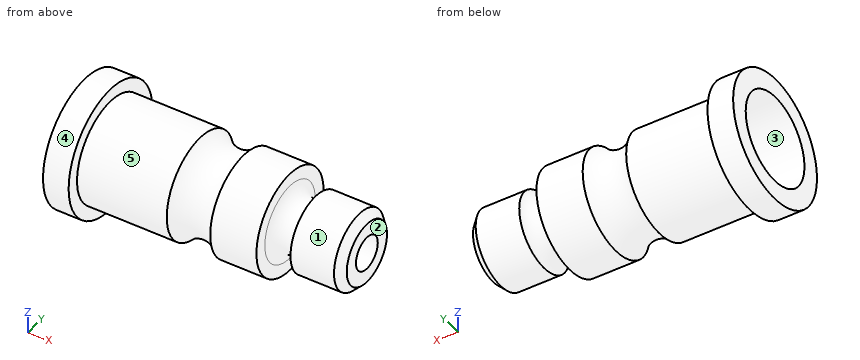
Autodesk Inventor part; units mm, degrees
ref_plane "YZ Plane" through (0, 0, 0) normal (1, 0, 0) x (0, 1, 0)
ref_plane "XZ Plane" through (0, 0, 0) normal (0, 1, 0) x (-1, 0, 0)
ref_plane "XY Plane" through (0, 0, 0) normal (0, 0, 1) x (1, 0, 0)
sketch "Skizze1" plane through (0, 0, 0) normal (0, 0, 1) x (1, 0, 0)
  line L0 (0, -1.0072) -> (0, 6.0435)
  line L1 (-2.2, 0) -> (13.2, 0)
  line L2 (0, 2.5) -> (0, 1.75)
  line L3 (0, 2.5) -> (1, 2.5)
  line L4 (1, 2.5) -> (1, 2)
  line L5 (1, 2) -> (4.5, 2)
  line L6 (0, 1.75) -> (4, 1.75)
  arc A0 (4.5, 2) -> (6.1971, 2) centre (5.3485, 2.7) ccw
  line L7 (6.1971, 2) -> (8, 2)
  line L8 (8, 2) -> (8, 1.5)
  arc A1 (8, 1.5) -> (9, 1.5) centre (8.5, 1.5) ccw
  line L9 (9, 1.5) -> (11, 1.5)
  line L10 (11, 1.5) -> (11, 0.65)
  line L11 (11, 0.65) -> (4.923, 0.65)
  line L12 (4.923, 0.65) -> (4, 1.75)
  line L13 (5.3485, 5.0362) -> (5.3485, 0.3638) construction
  point P0 (0, 0)
  dimension "d0" = 4
  dimension "d1" = 5
  dimension "d2" = 3.5
  dimension "d3" = 4
  dimension "d4" = 1.3
  dimension "d6" = 6.5
  dimension "d7" = 0.5
  dimension "d8" = 3
  dimension "d9" = 3
  dimension "d10" = 11
  dimension "d11" = 1
  dimension "d13" = 3.2
  dimension "d14" = 1.1
  dimension "d15" = 130
revolve "Umdrehung1" add sketch "Skizze1" angle 360 about axis through (-10, 0, 0) along (1, 0, 0)
thread "Gewinde1"
chamfer "Fase1" distance 0.3 angle 45 1 edges at (11, -1.5, 0)
properties part number "Öler"
Design review of the part built by this model. Coordinates are the model's own, in mm. Face numbers are marked on the shaded views. A direction names the side the tool comes from. Round coordinates to 2 decimals unless told otherwise and drop trailing zeros. Write each loop counter-clockwise with the first axis right and the second up, starting at its lowest first coordinate (ties: lowest second). Pieces come first, ordered by that corner, then holes.
Item 1: The part is to be moulded in two halves that separate along Z. For the marked faces 1, 2 and 3, say which applies: +Z half, -Z half, draft (parallel to the pull), parting line (faces both ways), or undercut.
Item 2: For the marked faces 4 and 5, list the 3-axis set-ups (+Z, -Z, +X, -X, +Y, -Y) from which the entire face can be reached by the end or side of a thin tool; tool diameter is ignored.
Item 3: We need section D-D on x = 9.5. Write out the cut boundary in (y, z), and give its area (3 significant figures).
Item 4: For probe 1 along Z at (x, y) = (1.4, 0); probe 2 along Z at (x, y) = (9.75, 0); probe 3 along X at (y, z) = (0.55, 2.15), list the stretches that pass through material, from the lowest coordinate up.
Item 5: Clearance check with flat-ended pins moving along their axes: pin 1 Ø2 at (x, z) = (3.5, 0.5) entering from -Y; pin 2 Ø1.5 at (x, y) = (3, 0) entering from -Z; pin 3 Ø2 at (y, z) = (0, 0) entering from -X. State where each tip first meets the part, or that it passes through.
Item 6: We need section A-A on y = 0. Write out the cut boundary in (x, z).
Item 7: We need section C-C on x = 7. Write out the cut boundary in (y, z), and give its area (3 significant figures).
Returned:
1. face 1: parting line
1. face 2: draft
1. face 3: undercut
2. face 4: +X, -X
2. face 5: +X
3. outline: circle Ø3 at (0, 0); hole circle Ø1.3 at (0, 0)
3. area: 5.74 mm2
4. probe 1: z = -2 to -1.75, 1.75 to 2
4. probe 2: z = -1.5 to -0.65, 0.65 to 1.5
4. probe 3: x = 0 to 1
5. pin 1: stops at y = -2
5. pin 2: stops at z = -2
5. pin 3: stops at x = 4.63
6. outline: (0, -2.5) - (1, -2.5) - (1, -2) - (4.5, -2) arc R1.1 cw to (6.2, -2) - (8, -2) - (8, -1.5) arc R0.5 cw to (9, -1.5) - (10.7, -1.5) - (11, -1.2) - (11, -0.65) - (4.92, -0.65) - (4, -1.75) - (0, -1.75) - close; (0, 1.75) - (4, 1.75) - (4.92, 0.65) - (11, 0.65) - (11, 1.2) - (10.7, 1.5) - (9, 1.5) arc R0.5 cw to (8, 1.5) - (8, 2) - (6.2, 2) arc R1.1 cw to (4.5, 2) - (1, 2) - (1, 2.5) - (0, 2.5) - close
7. outline: circle Ø4 at (0, 0); hole circle Ø1.3 at (0, 0)
7. area: 11.2 mm2
